Geometry: final body of the model. Coordinates: model frame, mm. A direction names the side the tool comes from. Round coordinates to 2 decimals unless told otherwise and drop trailing zeros. Loops run counter-clockwise (first coordinate to the right, second up) from the corner with the lowest first, then second, coordinate; pieces in that order, holes last. Notation, with made-up numbers: (44.25, 9) -> (61.25, 9) arc R25 cw to (61.25, 36) -> close; hole circle Ø6 at (4.5, -35.75). An arc over 180 degrees is marked (long way). Answer in a Markdown table with one row per item.
Autodesk Fusion 360 part; units mm, degrees
cylinder "CylinderPrimitive1" add diameter 18.542 height 26.924 placed x (1, 0, 0) y (0, 1, 0) z (0, 0, 1) at (0, 0, 0)
hole "Hole1" at (0, 0, 26.924) direction (0, 0, -1) diameter 10.7188 depth 14.986 tip angle 180
hole "Hole4" at (0, 0, 0) direction (0, 0, 1) diameter 10.7188 depth 11.43 tip angle 118
Item 1: First-contact query: P1, Ø1.5, axis at x = -1, y = 4, coming from the -Z side; P2, Ø5, axis at x = -6, z = 5, coming from the -Y side; P3, Ø2, axis at y = 2.5, z = 14.5, coming from the -X side; P4, Ø6.5, axis at x = 0, y = 0, coming from the -Z side. Flat tips, straight axial feed; report the tip coordinate or a pass-through.
Ans:
| item | result |
|---|---|
| P1 | z = 11.72 |
| P2 | y = -8.58 |
| P3 | x = -9.15 |
| P4 | through |
Item 2: Section query D-D, the plane y = 5.75. Output: boundary loops of the cut face in (x, z), and give its area (3 significant figures).
Ans:
| item | result |
|---|---|
| outline | (-7.27, 0) -> (7.27, 0) -> (7.27, 26.92) -> (-7.27, 26.92) -> close |
| area | 392 mm2 |
Item 3: Set-up query: faces 1 (the flat face through (4, -4, 26.924)), 2 (the cylindrical face through (-0.236, 5.354, 19.326)). Return all of +Z, -Z, +X, -X, +Y, -Y with unobstructed straight access to the full face (end or side cutting, diameter ignored); none if empty.
Ans:
| item | result |
|---|---|
| face 1 | +Z, +X, -X, +Y, -Y |
| face 2 | +Z |
Item 4: Ray query, L1, parallel to Y at x = 0, z = 20; L2, parallel to Y at x = -3, z = 7.25; L3, parallel to X at y = 4.25, z = 8.5. Return the intervals inside material, ascending.
Ans:
| item | result |
|---|---|
| L1 | -9.27 to -5.36, 5.36 to 9.27 |
| L2 | -8.77 to -4.44, 4.44 to 8.77 |
| L3 | -8.24 to -3.27, 3.27 to 8.24 |
Item 5: Section query A-A, the plane y = 0. Output: boundary loops of the cut face in (x, z).
Ans:
| item | result |
|---|---|
| outline | (-9.27, 0) -> (-5.36, 0) -> (-5.36, 11.43) -> (-4.51, 11.94) -> (-5.36, 11.94) -> (-5.36, 26.92) -> (-9.27, 26.92) -> close; (4.51, 11.94) -> (5.36, 11.43) -> (5.36, 0) -> (9.27, 0) -> (9.27, 26.92) -> (5.36, 26.92) -> (5.36, 11.94) -> close |
Item 6: Section query C-C, the plane z = 4. Output: boundary loops of the cut face in (x, y), and give its area (3 significant figures).
Ans:
| item | result |
|---|---|
| outline | circle Ø18.54 at (0, 0); hole circle Ø10.72 at (0, 0) |
| area | 180 mm2 |
Item 7: Mould query, pull axis Y, two halves, no side actions, for faces 3 (the cylindrical face through (-6.8, 6.3, 13.7)), 4 (the cylindrical face through (-0.236, -5.354, 5.795)), 5 (the flat face through (4, -4, 0)), 6 (the flat face through (4, 3, 11.938)). Classes: released by +Y, released by -Y, zero draft, split by the parting line, or undercut.
Ans:
| item | result |
|---|---|
| face 3 | split by the parting line |
| face 4 | undercut |
| face 5 | zero draft |
| face 6 | undercut |
